from build123d import *

# Parameters (mm, degrees)
BOSS_EXTRUDE1_DEPTH = 26
SKETCH2_R           = 1.7
CUT_EXTRUDE1_DEPTH  = 31
CUT_EXTRUDE2_DEPTH  = 1


with BuildPart() as part:
    # Sketch1 → Boss-Extrude1 (new body)
    with BuildSketch(Plane(origin=(0, 0, 0), x_dir=(1, 0, 0), z_dir=(0, 1, 0))):
        with BuildLine():
            Line((-46.998275301, 32.528571429), (-46.998275301, -39.471428571))
            Line((-46.998275301, -39.471428571), (-16.998275301, -39.471428571))
            Line((-16.998275301, -39.471428571), (-16.998275301, -28.471428571))
            ThreePointArc((-16.998275301, -28.471428571), (-41.998275301, -3.471428571), (-16.998275301, 21.528571429))
            Line((-16.998275301, 21.528571429), (-16.998275301, 32.528571429))
            Line((-16.998275301, 32.528571429), (-46.998275301, 32.528571429))
        make_face()
    extrude(amount=BOSS_EXTRUDE1_DEPTH)

    # Sketch2 → Cut-Extrude1 (cut, through all)
    with BuildSketch(Plane(origin=(-16.998275301, 0, 0), x_dir=(0, 0, -1), z_dir=(1, 0, 0))):
        with Locations((-34.471428571, 13)):
            Circle(SKETCH2_R)
        with Locations((27.528571429, 13)):
            Circle(SKETCH2_R)
    extrude(amount=-CUT_EXTRUDE1_DEPTH, mode=Mode.SUBTRACT)

    # Sketch3 → Cut-Extrude2 (cut)
    with BuildSketch(Plane(origin=(-16.998275301, 0, 0), x_dir=(0, 0, -1), z_dir=(1, 0, 0))):
        Polygon((-34.164231178, 21.664809495), (-32.617436306, 21.664809495), (-32.617436306, 21.33916847), (-33.87929528, 21.33916847), (-33.87929528, 20.362245393), (-32.617436306, 20.362245393), (-32.617436306, 20.036604367), (-33.87929528, 20.036604367), (-33.87929528, 18.489809495), (-34.164231178, 18.489809495), align=None)
        with BuildLine():
            Line((-30.867115793, 21.746219752), (-30.647053694, 21.573858975))
            Line((-30.647053694, 21.573858975), (-31.485960945, 20.291011418))
            add(Edge.make_bspline(
                [(-31.485960945, 20.291011418), (-31.430107908, 20.299913992), (-31.321160245, 20.317279468), (-31.210882608, 20.320144176), (-31.157139832, 20.321540265)],
                knots=[0, 0, 0, 0, 0.000169463, 0.000330556, 0.000330556, 0.000330556, 0.000330556], degree=3))
            add(Edge.make_bspline(
                [(-31.157139832, 20.321540265), (-31.124868872, 20.320685496), (-31.061554556, 20.319008476), (-30.968523034, 20.3057555), (-30.879108327, 20.285127316), (-30.793509908, 20.254936716), (-30.711619139, 20.216383115), (-30.632967755, 20.170173711), (-30.559033768, 20.113925858), (-30.488865205, 20.051092605), (-30.425159193, 19.981499352), (-30.368756629, 19.907656708), (-30.321379468, 19.829641624), (-30.282940267, 19.747493609), (-30.253090842, 19.661339295), (-30.231330621, 19.571288912), (-30.218467705, 19.477280362), (-30.216721009, 19.413346589), (-30.215833742, 19.380870192)],
                knots=[0, 0, 0, 0, 9.6777e-05, 0.000189873, 0.000281356, 0.000371672, 0.000461583, 0.000552553, 0.000644776, 0.000739798, 0.000834778, 0.000927384, 0.001018136, 0.001108046, 0.001198964, 0.001291213, 0.001385568, 0.001482981, 0.001482981, 0.001482981, 0.001482981], degree=3))
            add(Edge.make_bspline(
                [(-30.215833742, 19.380870192), (-30.217124701, 19.336438604), (-30.219665004, 19.249007753), (-30.244977733, 19.121666026), (-30.284311125, 19.00035153), (-30.340533597, 18.887001153), (-30.410367616, 18.781770251), (-30.495528004, 18.68852915), (-30.592994597, 18.60537133), (-30.703200478, 18.535832826), (-30.821803024, 18.479042915), (-30.946400908, 18.438253017), (-31.075784105, 18.413140155), (-31.163599713, 18.409991823), (-31.208021242, 18.408399239)],
                knots=[0, 0, 0, 0, 0.000133147, 0.000262001, 0.000387907, 0.000514768, 0.000640365, 0.000765549, 0.000892346, 0.001023614, 0.001155333, 0.001285865, 0.00141597, 0.001549154, 0.001549154, 0.001549154, 0.001549154], degree=3))
            add(Edge.make_bspline(
                [(-31.208021242, 18.408399239), (-31.250744677, 18.40978554), (-31.335372323, 18.412531559), (-31.459862072, 18.436993517), (-31.579480666, 18.476642103), (-31.693390033, 18.531265056), (-31.798909447, 18.600260421), (-31.893311845, 18.683320489), (-31.976126527, 18.778669789), (-32.045046361, 18.886293533), (-32.09970964, 19.001945137), (-32.140703357, 19.122538129), (-32.164648521, 19.247633112), (-32.167994569, 19.33243386), (-32.169679896, 19.375146034)],
                knots=[0, 0, 0, 0, 0.000128067, 0.000253679, 0.000378981, 0.000505286, 0.000631591, 0.000755981, 0.000881329, 0.001009234, 0.001138109, 0.001264215, 0.001390451, 0.001518558, 0.001518558, 0.001518558, 0.001518558], degree=3))
            add(Edge.make_bspline(
                [(-32.169679896, 19.375146034), (-32.168608156, 19.40784362), (-32.166419869, 19.474605844), (-32.151140508, 19.57571964), (-32.126588873, 19.679180265), (-32.099093149, 19.76695014), (-32.070041346, 19.838851664), (-32.045863685, 19.896821259), (-32.015770131, 19.956475947), (-31.983681421, 20.019861316), (-31.946709119, 20.085343816), (-31.906508494, 20.154017859), (-31.861968096, 20.224791265), (-31.830744092, 20.272819213), (-31.814782059, 20.297371595)],
                knots=[0, 0, 0, 0, 9.8079e-05, 0.000200258, 0.00030609, 0.000416919, 0.000475736, 0.000538705, 0.000605266, 0.000676095, 0.000751832, 0.000830806, 0.000914808, 0.001002664, 0.001002664, 0.001002664, 0.001002664], degree=3))
            Line((-31.814782059, 20.297371595), (-30.867115793, 21.746219752))
        make_face()
        with BuildLine():
            add(Edge.make_bspline(
                [(-31.216925489, 19.995899239), (-31.24111118, 19.995184076), (-31.288563308, 19.993780933), (-31.358094863, 19.985856379), (-31.423723348, 19.970840263), (-31.48620269, 19.95142058), (-31.544865998, 19.924964542), (-31.600440512, 19.893262694), (-31.652286601, 19.855281097), (-31.700151178, 19.812404161), (-31.743525509, 19.765416612), (-31.780883963, 19.71510002), (-31.813107522, 19.662653711), (-31.839307545, 19.607642956), (-31.859709233, 19.550087877), (-31.874466867, 19.490253426), (-31.882679911, 19.427738302), (-31.884046278, 19.385345247), (-31.884743998, 19.363697717)],
                knots=[0, 0, 0, 0, 7.2576e-05, 0.000142393, 0.000209516, 0.000274284, 0.000338345, 0.000402166, 0.000465901, 0.000530762, 0.000594681, 0.000657393, 0.000718477, 0.000779073, 0.000839825, 0.000901374, 0.000963619, 0.001028571, 0.001028571, 0.001028571, 0.001028571], degree=3))
            add(Edge.make_bspline(
                [(-31.884743998, 19.363697717), (-31.884175799, 19.342243806), (-31.883061645, 19.300175882), (-31.872944897, 19.238182483), (-31.857491644, 19.178524316), (-31.834504285, 19.121508938), (-31.807084179, 19.066267278), (-31.770884349, 19.014800269), (-31.730773408, 18.963982062), (-31.68282734, 18.917716442), (-31.631371146, 18.874666504), (-31.576397198, 18.837037988), (-31.519102092, 18.80484696), (-31.458712302, 18.779618321), (-31.396084625, 18.758913432), (-31.330697265, 18.744343376), (-31.262504746, 18.736106042), (-31.216311274, 18.734737895), (-31.192756819, 18.734040265)],
                knots=[0, 0, 0, 0, 6.4316e-05, 0.000126115, 0.000187979, 0.000248804, 0.000310245, 0.000372516, 0.000437181, 0.000504193, 0.000571946, 0.000638278, 0.00070376, 0.000768733, 0.000834302, 0.000901425, 0.000969348, 0.001040017, 0.001040017, 0.001040017, 0.001040017], degree=3))
            add(Edge.make_bspline(
                [(-31.192756819, 18.734040265), (-31.169202402, 18.734737949), (-31.123009006, 18.736106204), (-31.054815938, 18.744342761), (-30.989430606, 18.758915691), (-30.926795559, 18.779610133), (-30.866432975, 18.804877336), (-30.809187978, 18.83683772), (-30.754733922, 18.874897913), (-30.703243949, 18.917642872), (-30.655497448, 18.964245388), (-30.614424488, 19.014346636), (-30.579333269, 19.066683241), (-30.550817971, 19.121291327), (-30.528083799, 19.178558791), (-30.512552183, 19.238173248), (-30.502456328, 19.3001783), (-30.501339303, 19.342244623), (-30.500769639, 19.363697717)],
                knots=[0, 0, 0, 0, 7.067e-05, 0.000138593, 0.000205716, 0.000271284, 0.000336258, 0.00040174, 0.000467548, 0.000535301, 0.000602313, 0.00066738, 0.000729296, 0.000791029, 0.000851854, 0.000913718, 0.000975517, 0.001039833, 0.001039833, 0.001039833, 0.001039833], degree=3))
            add(Edge.make_bspline(
                [(-30.500769639, 19.363697717), (-30.501268834, 19.385373487), (-30.502248592, 19.427915974), (-30.513330193, 19.490225471), (-30.52869938, 19.550391855), (-30.551906718, 19.608037305), (-30.582057489, 19.662933151), (-30.618779885, 19.715361265), (-30.661270923, 19.765705799), (-30.710317034, 19.812524596), (-30.763707476, 19.85501674), (-30.820114642, 19.893405283), (-30.879889589, 19.92466945), (-30.941953816, 19.951510565), (-31.007054871, 19.970532437), (-31.074481667, 19.985903262), (-31.144873114, 19.993714686), (-31.192741951, 19.995166019), (-31.216925489, 19.995899239)],
                knots=[0, 0, 0, 0, 6.4952e-05, 0.000127479, 0.000189343, 0.000250994, 0.000313327, 0.000376843, 0.000442725, 0.000510648, 0.000579881, 0.000647266, 0.000714983, 0.000781961, 0.000849765, 0.00091813, 0.000989211, 0.001061786, 0.001061786, 0.001061786, 0.001061786], degree=3))
        make_face(mode=Mode.SUBTRACT)
    extrude(amount=-CUT_EXTRUDE2_DEPTH, mode=Mode.SUBTRACT)


solid = part.part
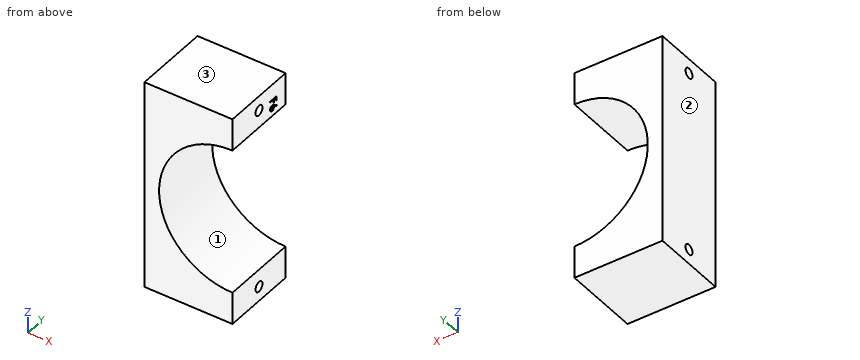
The listing builds one solid part. Answer for the finished solid, in the listing's coordinates (mm). Face numbers are marked on the shaded views. Give positions to 0.01 mm unless a question says otherwise; leave off trailing zeros. Order: outer loops, then holes, each group sorted by start corner. A loop starts at its lowest first (then second) coordinate and runs counter-clockwise, first axis right, second up. Notation, with made-up numbers: (-36.5, 89.5) - (-16.5, 89.5) arc R20 ccw to (-16.5, 112.5) - close; hole circle Ø10 at (75.5, -35). An arc over 180 degrees is marked (long way). One line per item, written item: value. Start each with the question number.
1) Given pin 1 Ø8 at (x, z) = (-34, 13) entering from -Y, flat-ended and moving along its own axis, determine where the tip first touches the part or whether it passes through.
2) The mould has two halves that part along Z. Classify the marked faces 1, 2 and 3: released by +Z, released by -Z, zero draft, split by the parting line, or undercut.
3) A cutting plane is placed at D-D on y = 17.75. Give the vertices of the cut face in (x, z).
4) A cutting plane is placed at A-A on y = 13. Give the vertices of the cut face in (x, z), then the cut area to 3 significant figures.
5) A cutting plane is placed at C-C on x = -21.5. Give the vertices of the cut face in (y, z), then the cut area to 3 significant figures.
6) A cutting plane is placed at B-B on x = -26.5. Give the vertices of the cut face in (y, z), then the cut area to 3 significant figures.
7) Find the intervals of material crossed by L1, parallel to Z at x = -18.5, y = 12; L2, parallel to Z at x = -40, y = 24.25; L3, parallel to Z at x = -29.5, y = 23.5, in increasing order.
Answer sheet:
1. pin 1: passes through
2. face 1: undercut
2. face 2: zero draft
2. face 3: released by +Z
3. outline: (-47, -32.53) - (-17, -32.53) - (-17, -21.53) arc R25 cw to (-17, 28.47) - (-17, 39.47) - (-47, 39.47) - close
4. outline: (-47, -32.53) - (-17, -32.53) - (-17, -29.23) - (-47, -29.23) - close; (-47, -25.83) - (-17, -25.83) - (-17, -21.53) arc R25 cw to (-17, 28.47) - (-17, 32.77) - (-47, 32.77) - close; (-47, 36.17) - (-17, 36.17) - (-17, 39.47) - (-47, 39.47) - close
4. area: 974 mm2
5. outline: (0, -32.53) - (26, -32.53) - (26, -21.12) - (0, -21.12) - close; (0, 28.06) - (26, 28.06) - (26, 39.47) - (0, 39.47) - close; hole circle Ø3.4 at (13, -27.53); hole circle Ø3.4 at (13, 34.47)
5. area: 575 mm2
6. outline: (0, -32.53) - (26, -32.53) - (26, -19.65) - (0, -19.65) - close; (0, 26.6) - (26, 26.6) - (26, 39.47) - (0, 39.47) - close; hole circle Ø3.4 at (13, -27.53); hole circle Ø3.4 at (13, 34.47)
6. area: 651 mm2
7. L1: z = -32.53 to -28.9, -26.15 to -21.48, 28.43 to 33.1, 35.85 to 39.47
7. L2: z = -32.53 to -6.32, 13.27 to 39.47
7. L3: z = -32.53 to -18.18, 25.12 to 39.47
